Read the model definition and answer for the solid it produces. Units are mm, in the model's axes. A direction names the side the tool comes from. Give positions to 0.01 mm unless a question says otherwise; leave off trailing zeros. Loops run counter-clockwise (first coordinate to the right, second up) from the corner with the lowest first, then second, coordinate; pieces in that order, holes last. Notation, with made-up numbers: (-3.75, 56.5) - (22.25, 56.5) arc R22 ccw to (22.25, 72.5) - close; hole circle Ø10 at (16.5, 28.5). An arc over 180 degrees is marked (long way). Use a Markdown table: item, result. Add a question column.
Item 1: Consider probe 1 along Y at (x, z) = (-15, 0.85); probe 2 along Y at (x, z) = (0, 0.7); probe 3 along X at (y, z) = (23.5, -0.7). Determine where each line is inside the solid, lowest interval first. Write a range as [from, to].
Item 2: For a pull along Y with two mould halves and no side action, classify faces 1 (the face through (15, 0, 0)), 2 (the face through (-15, 23, 0)), 3 (the face through (0, 3, 2.5)) as +Y half, -Y half, draft (parallel to the pull), parting line (faces both ways), or undercut.
Item 3: A cutting plane is placed at A-A (x = -15). Determine the outline of the cut face in (y, z), plus the area to 3 significant figures.
Item 4: Each of these flat-tipped pins is pushed along its axis until it touches: P1, Ø1.5, axis at y = -28, z = 0, coming from the +X side; P2, Ø3, axis at y = -17, z = -1.5, coming from the -X side; P3, Ø2.5, axis at x = -13, z = 0, coming from the -Y side. Where does it stop, or does it pass through?
Item 5: A cutting plane is placed at D-D (y = -25). Determine the outline of the cut face in (x, z), plus the area to 3 significant figures.
Item 6: A cutting plane is placed at C-C (z = -1.8). Determine the outline of the cut face in (x, y), plus the area to 3 significant figures.
Item 7: A cutting plane is placed at B-B (y = 5). Determine the outline of the cut face in (x, z), plus the area to 3 significant figures.
Item 8: Which of the six approach directions +Z, -Z, +X, -X, +Y, -Y give full straight-line access (tool end or side, diameter ignored) to faces 4 (the face through (13, 5, 0)), 5 (the face through (10, -20, 0)), 6 (the face through (-10, -20, 0))?
from build123d import *

# Parameters (mm, degrees)
BOSS_EXTRUDE1_DEPTH = 2.5
SKETCH2_R           = 2.5
SKETCH2_R_2         = 4
CUT_EXTRUDE1_DEPTH  = 46
SKETCH3_R           = 2
CUT_EXTRUDE2_DEPTH  = 10


with BuildPart() as part:
    # Sketch1 → Boss-Extrude1 (new, symmetric)
    with BuildSketch(Plane.XY):
        Polygon((-20, 30), (-20, 0), (-10, 0), (-10, -40), (10, -40), (10, 0), (20, 0), (20, 30), align=None)
    extrude(amount=BOSS_EXTRUDE1_DEPTH, both=True)

    # Sketch2 → Cut-Extrude1 (cut, through all)
    with BuildSketch(Plane.XY.offset(2.5)):
        with Locations((-25, 20)):
            Circle(SKETCH2_R)
        with Locations((25, 20)):
            Circle(SKETCH2_R)
        with Locations((0, -25)):
            Circle(SKETCH2_R_2)
    extrude(amount=-CUT_EXTRUDE1_DEPTH, mode=Mode.SUBTRACT)

    # Sketch3 → Cut-Extrude2 (cut)
    with BuildSketch(Plane.XY.offset(2.5)):
        with Locations((-15, 25)):
            Circle(SKETCH3_R)
        with Locations((15, 25)):
            Circle(SKETCH3_R)
        with Locations((15, 5)):
            Circle(SKETCH3_R)
        with Locations((-15, 5)):
            Circle(SKETCH3_R)
    extrude(amount=-CUT_EXTRUDE2_DEPTH, mode=Mode.SUBTRACT)


solid = part.part
Geometry says:
| question | item | result |
|---|---|---|
| 1 | probe 1 | [0, 3], [7, 23], [27, 30] |
| 1 | probe 2 | [-40, -29], [-21, 30] |
| 1 | probe 3 | [-20, -16.32], [-13.68, 13.68], [16.32, 20] |
| 2 | face 1 | -Y half |
| 2 | face 2 | undercut |
| 2 | face 3 | draft |
| 3 | outline | (0, -2.5) - (3, -2.5) - (3, 2.5) - (0, 2.5) - close; (7, -2.5) - (23, -2.5) - (23, 2.5) - (7, 2.5) - close; (27, -2.5) - (30, -2.5) - (30, 2.5) - (27, 2.5) - close |
| 3 | area | 110 mm² |
| 4 | P1 | x = 10 |
| 4 | P2 | x = -10 |
| 4 | P3 | y = 0 |
| 5 | outline | (-10, -2.5) - (-4, -2.5) - (-4, 2.5) - (-10, 2.5) - close; (4, -2.5) - (10, -2.5) - (10, 2.5) - (4, 2.5) - close |
| 5 | area | 60.0 mm² |
| 6 | outline | (-20, 0) - (-10, 0) - (-10, -40) - (10, -40) - (10, 0) - (20, 0) - (20, 30) - (-20, 30) - close; hole circle Ø4 at (-15, 5); hole circle Ø4 at (-15, 25); hole circle Ø8 at (0, -25); hole circle Ø4 at (15, 5); hole circle Ø4 at (15, 25) |
| 6 | area | 1,900 mm² |
| 7 | outline | (-20, -2.5) - (-17, -2.5) - (-17, 2.5) - (-20, 2.5) - close; (-13, -2.5) - (13, -2.5) - (13, 2.5) - (-13, 2.5) - close; (17, -2.5) - (20, -2.5) - (20, 2.5) - (17, 2.5) - close |
| 7 | area | 160 mm² |
| 8 | face 4 | +Z, -Z |
| 8 | face 5 | +Z, -Z, +X, -Y |
| 8 | face 6 | +Z, -Z, -X, -Y |
